Build history of the part. All positions in model axes, mm. Face numbers are marked on the shaded views. Round coordinates to 2 decimals unless told otherwise and drop trailing zeros. Order: outer loops, then holes, each group sorted by start corner. A loop starts at its lowest first (then second) coordinate and runs counter-clockwise, first axis right, second up. Notation, with made-up numbers: (45.5, 78.5) -> (98.5, 78.5) arc R19 ccw to (98.5, 90.5) -> close; hole circle Ø4 at (4, 65). An arc over 180 degrees is marked (long way). Answer as CSV lines item,"result". Start each with the question number.
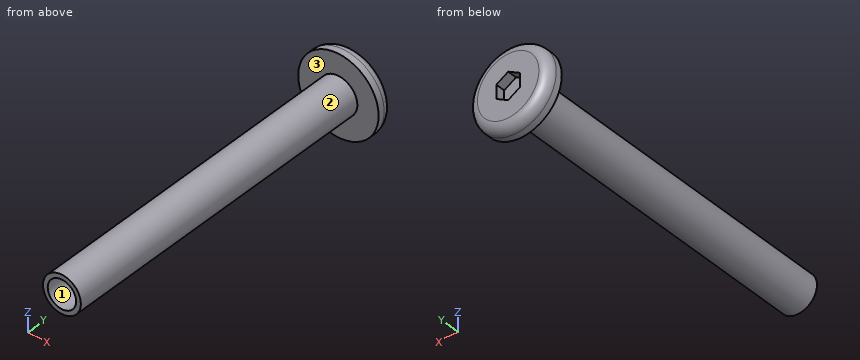
```python
from build123d import *

# Parameters (mm, degrees)
SKETCH_1_R          = 2
SKETCH_1_R_2        = 1.5
EXTRUDE_1_DEPTH     = 35
SKETCH_2_R          = 4.25
EXTRUDE_2_DEPTH     = 1.7
CUT_EXTRUDE_1_DEPTH = 1
FILLET_1_R          = 1


with BuildPart() as part:
    # 草图1 → 凸台-拉伸1 (new body)
    with BuildSketch(Plane(origin=(0, 0, 0), x_dir=(1, 0, 0), z_dir=(0, 1, 0))):
        with Locations(Location((0, 0, 0), (0, 0, 270))):
            Circle(SKETCH_1_R)
        with Locations(Location((0, 0, 0), (0, 0, 270))):
            Circle(SKETCH_1_R_2, mode=Mode.SUBTRACT)
    extrude(amount=EXTRUDE_1_DEPTH)

    # 草图2 → 凸台-拉伸2 (add)
    with BuildSketch(Plane(origin=(0, 35, 0), x_dir=(1, 0, 0), z_dir=(0, 1, 0))):
        with Locations(Location((0, 0, 0), (0, 0, 270))):
            Circle(SKETCH_2_R)
    extrude(amount=EXTRUDE_2_DEPTH)

    # 草图3 → 切除-拉伸1 (cut)
    with BuildSketch(Plane(origin=(0, 36.7, 0), x_dir=(1, 0, 0), z_dir=(0, 1, 0))):
        Polygon((1.25, 0.721687836), (0, 1.443375673), (-1.25, 0.721687836), (-1.25, -0.721687836), (0, -1.443375673), (1.25, -0.721687836), align=None)
    extrude(amount=-CUT_EXTRUDE_1_DEPTH, mode=Mode.SUBTRACT)

    # 圆角1
    fillet_1_edges = [part.edges().sort_by_distance(p)[0] for p in [
        (0, 36.7, -4.25),
    ]]
    fillet(fillet_1_edges, radius=FILLET_1_R)


solid = part.part
```
Q1. Two-plate mould, pull along Z, no slides. Class the marked faces 1, 2 and 3: +Z half, -Z half, draft (parallel to the pull), parting line (faces both ways), or undercut.
Q2. Probe L1, parallel to X at y = 27, z = 0; L2, parallel to Y at x = -3, z = 0.75; L3, parallel to Y at x = 0, z = 0. List the from-to ranges inside material, lowest first.
Q3. Slice it at B-B, the plane y = 7. Write the cut outline in (x, z).
Q4. Flat gauge pins, fed straight in: pin 1 Ø0.9 at (x, z) = (0.5, 0) entering from -Y; pin 2 Ø1.5 at (x, y) = (1, 12.5) entering from +Z; pin 3 Ø1.5 at (y, z) = (13.5, 1.5) entering from +X. Where does each tip first touch, or does it go through?
Q5. Slice it at A-A, the plane z = 0. Write the cut outline in (x, y).
Solutions:
1,face 1,"undercut"
1,face 2,"parting line"
1,face 3,"draft"
2,L1,"x = -2 to -1.5, 1.5 to 2"
2,L2,"y = 35 to 36.7"
2,L3,"y = 35 to 35.7"
3,outline,"circle Ø4 at (0, 0); hole circle Ø3 at (0, 0)"
4,pin 1,"stops at y = 35"
4,pin 2,"stops at z = 1.98"
4,pin 3,"stops at x = 1.85"
5,outline,"(-4.25, 35) -> (-2, 35) -> (-2, 0) -> (-1.5, 0) -> (-1.5, 35) -> (1.5, 35) -> (1.5, 0) -> (2, 0) -> (2, 35) -> (4.25, 35) -> (4.25, 35.7) arc R1 ccw to (3.25, 36.7) -> (1.25, 36.7) -> (1.25, 35.7) -> (-1.25, 35.7) -> (-1.25, 36.7) -> (-3.25, 36.7) arc R1 ccw to (-4.25, 35.7) -> close"
